Autodesk Fusion 360 part; units mm, degrees
sketch "Sketch1" plane through (0, 0, 0) normal (0, 0, 1) x (1, 0, 0)
  line L0 (45, 34.5) -> (-40, 34.5)
  line L1 (-40, 34.5) -> (-40, -34.5)
  line L2 (-40, -34.5) -> (45, -34.5)
  line L3 (45, -34.5) -> (45, 34.5)
  circle A0 centre (41, 30.9952) radius 1.5
  line L4 (0, 56) -> (0, -61) construction
  line L5 (-71, -0.0048) -> (62, -0.0048) construction
  circle A1 centre (41, 30.9952) radius 2.5
  circle A2 centre (-36, 30.9952) radius 1.5
  circle A3 centre (-36, 30.9952) radius 2.5
  circle A4 centre (41, -31.0048) radius 1.5
  circle A5 centre (41, -31.0048) radius 2.5
  circle A6 centre (-36, -31.0048) radius 1.5
  circle A7 centre (-36, -31.0048) radius 2.5
  circle A8 centre (36, 24.4952) radius 1.25
  circle A9 centre (-22, 24.4952) radius 1.25
  circle A10 centre (36, -24.5048) radius 1.25
  circle A11 centre (-22, -24.5048) radius 1.25
  dimension "d1" = 85
  dimension "d2" = 69
  dimension "d3" = 3
  dimension "d8" = 5
  dimension "d13" = 2.5
  dimension "d14" = 24.5
  dimension "d17" = -58
  dimension "d18" = -49
  dimension "d45" = 41
  dimension "d46" = 41
  dimension "d47" = 41
extrude "Extrude1" add sketch "Sketch1" against normal blind 1.5 contours L0 L1 L2 L3 | A1 | A3 | A5 | A7
extrude "Extrude2" add sketch "Sketch1" along normal blind 4 contours L0 L1 L2 L3
fillet "Fillet1" radius 2 4 edges at (-40, -34.5, 1.25) (45, -34.5, 1.25) (45, 34.5, 1.25) (-40, 34.5, 1.25)
sketch "Sketch2" plane through (0, 0, 4) normal (0, 0, 1) x (-1, 0, 0)
  circle A0 centre (22, 24.5048) radius 1.25
  circle A1 centre (22, -24.4952) radius 1.25
  circle A2 centre (-36, 24.5048) radius 1.25
  circle A3 centre (-41, 31.0048) radius 2.5
  circle A4 centre (36, -30.9952) radius 2.5
  circle A5 centre (-36, -24.4952) radius 1.25
  circle A6 centre (36, 31.0048) radius 2.5
  circle A7 centre (-41, -30.9952) radius 2.5
  arc A8 (38, -34.5) -> (40, -32.5) centre (38, -32.5) ccw
  line L0 (40, -32.5) -> (40, 32.5)
  arc A9 (40, 32.5) -> (38, 34.5) centre (38, 32.5) ccw
  line L1 (38, 34.5) -> (-43, 34.5)
  arc A10 (-43, 34.5) -> (-45, 32.5) centre (-43, 32.5) ccw
  line L2 (-45, 32.5) -> (-45, -32.5)
  arc A11 (-45, -32.5) -> (-43, -34.5) centre (-43, -32.5) ccw
  line L3 (-43, -34.5) -> (38, -34.5)
  line L4 (34, -20.4952) -> (-37, -20.4952)
  line L5 (-37, -20.4952) -> (-37, 20.5048)
  line L6 (-37, 20.5048) -> (34, 20.5048)
  line L7 (34, 20.5048) -> (34, -20.4952)
  dimension "d28" = 4
  dimension "d29" = 6
  dimension "d30" = 8
extrude "Extrude3" cut sketch "Sketch2" against normal blind 5.5 contours L4 L5 L6 L7
fillet "Fillet2" radius 2 4 edges at (-34, 20.4952, 1.25) (-34, -20.5048, 1.25) (37, -20.5048, 1.25) (37, 20.4952, 1.25)
sketch "Sketch3" plane through (0, 0, 4) normal (0, 0, 1) x (-1, 0, 0)
  line L0 (-37, -18.4952) -> (-37, 18.5048)
  arc A0 (-35, 20.5048) -> (-37, 18.5048) centre (-35, 18.5048) ccw
  line L1 (-35, 20.5048) -> (32, 20.5048)
  arc A1 (34, 18.5048) -> (32, 20.5048) centre (32, 18.5048) ccw
  line L2 (34, 18.5048) -> (34, -18.4952)
  arc A2 (32, -20.4952) -> (34, -18.4952) centre (32, -18.4952) ccw
  line L3 (32, -20.4952) -> (-35, -20.4952)
  arc A3 (-37, -18.4952) -> (-35, -20.4952) centre (-35, -18.4952) ccw
  circle A4 centre (22, 24.5048) radius 1.25
  circle A5 centre (22, -24.4952) radius 1.25
  circle A6 centre (-36, 24.5048) radius 1.25
  circle A7 centre (-41, 31.0048) radius 2.5
  circle A8 centre (36, -30.9952) radius 2.5
  circle A9 centre (-36, -24.4952) radius 1.25
  circle A10 centre (36, 31.0048) radius 2.5
  circle A11 centre (-41, -30.9952) radius 2.5
  arc A12 (38, -34.5) -> (40, -32.5) centre (38, -32.5) ccw
  line L4 (40, -32.5) -> (40, 32.5)
  arc A13 (40, 32.5) -> (38, 34.5) centre (38, 32.5) ccw
  line L5 (38, 34.5) -> (-43, 34.5)
  arc A14 (-43, 34.5) -> (-45, 32.5) centre (-43, 32.5) ccw
  line L6 (-45, 32.5) -> (-45, -32.5)
  arc A15 (-45, -32.5) -> (-43, -34.5) centre (-43, -32.5) ccw
  line L7 (-43, -34.5) -> (38, -34.5)
  circle A16 centre (22, -24.4952) radius 3
  circle A17 centre (-36, -24.4952) radius 3
  circle A18 centre (22, 24.5048) radius 3
  circle A19 centre (-36, 24.5048) radius 3
  dimension "d35" = 6
  dimension "d38" = -58
  dimension "d39" = 49
extrude "Extrude4" add sketch "Sketch3" along normal blind 2.5 contours A16 | A17 | A18 | A19
equation "d46 = d45"
equation "d47 = d45"
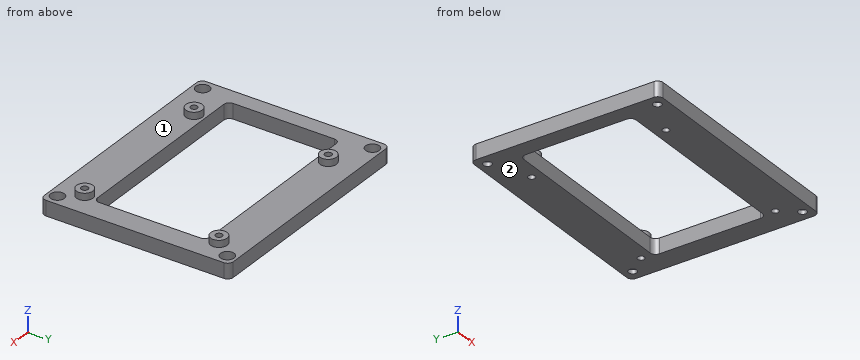
Work out the finished part from the listing and answer in its coordinate system (mm). Face numbers are marked on the shaded views. Coordinates: 2 decimals unless noted, no trailing zeros. Loops run counter-clockwise (first coordinate to the right, second up) from the corner with the lowest first, then second, coordinate; pieces in that order, holes last. Notation, with made-up numbers: M 34.25,-21.75 L 56.25,-21.75 A31 cw 56.25,4.25 Z; hole C -33,-29 d11. An arc over 180 degrees is marked long. Use CSV: the item, a comma, the result in double quotes. Start each with the question number.
(1) Given pin 1 Ø2.5 at (x, y) = (-36.5, 31) entering from +Z; pin 2 Ø5.5 at (x, y) = (41.5, -31) entering from +Z, each flat-ended and moving along its own axis, determine where each tip first touches the part or whether it passes through.
(2) Find section C-C, the plane y = -13.5. Give the vertices of the cut face in (x, z), then the cut area to 3 significant figures.
(3) Find section A-A, the plane z = 5. Give the vertices of the cut face in (x, y).
(4) Consider line 1 (Y direction, x = 36, z = 5); line 2 (Y direction, x = 41, z = -1); line 3 (Y direction, x = -36, z = 2.25). Determine where each line is inside the solid, lowest interval first.
(5) Find section B-B, the plane x = -11.5. Give the vertices of the cut face in (y, z).
(6) For a pull along X with two mould halves and no side action, classify the marked faces 1 and 2 as +X half, -X half, draft (parallel to the pull), parting line (faces both ways), or undercut.
(7) Find section D-D, the plane x = 41. Give the vertices of the cut face in (y, z).
Recorded:
1,pin 1,"stops at z = 0"
1,pin 2,"stops at z = 4"
2,outline,"M -40,-1.5 L -34,-1.5 L -34,4 L -40,4 Z; M 37,-1.5 L 45,-1.5 L 45,4 L 37,4 Z"
2,area,"77.0 mm^2"
3,outline,"C -22,-24.5 d6; C -22,24.5 d6; C 36,-24.5 d6; C 36,24.5 d6; hole C -22,-24.5 d2.5; hole C -22,24.5 d2.5; hole C 36,-24.5 d2.5; hole C 36,24.5 d2.5"
4,line 1,"y = -27.5 to -25.75, -23.25 to -21.5, 21.5 to 23.25, 25.75 to 27.5"
4,line 2,"y = -34.5 to -32.5, -29.5 to 29.5, 32.5 to 34.5"
4,line 3,"y = -34.5 to -33.5, -28.5 to 28.5, 33.5 to 34.5"
5,outline,"M -34.5,-1.5 L -20.5,-1.5 L -20.5,4 L -34.5,4 Z; M 20.5,-1.5 L 34.5,-1.5 L 34.5,4 L 20.5,4 Z"
6,face 1,"undercut"
6,face 2,"draft"
7,outline,"M -34.5,-1.5 L -32.5,-1.5 L -32.5,0 L -33.5,0 L -33.5,4 L -34.5,4 Z; M -29.5,-1.5 L 29.5,-1.5 L 29.5,0 L 28.5,0 L 28.5,4 L -28.5,4 L -28.5,0 L -29.5,0 Z; M 32.5,-1.5 L 34.5,-1.5 L 34.5,4 L 33.5,4 L 33.5,0 L 32.5,0 Z"
